Can you work these out from the model? Positions are in its coordinate system, mm. Round coordinates to 2 decimals unless told otherwise and drop trailing zeros. Loops run counter-clockwise (first coordinate to the right, second up) from the corner with the lowest first, then second, coordinate; pieces in that order, holes last. Notation, with made-up numbers: (42.25, 65.25) -> (63.25, 65.25) arc R12 ccw to (63.25, 81.25) -> close; hole circle Ø8 at (74.25, 36). An arc over 180 degrees is marked (long way). Use a Markdown table: item, result.
from build123d import *

# Parameters (mm, degrees)
SKETCH1_W           = 3.175
SKETCH1_H           = 7.62
BOSS_EXTRUDE1_DEPTH = 1.5875


with BuildPart() as part:
    # Sketch1 → Boss-Extrude1 (new body)
    with BuildSketch(Plane.XY):
        Polygon((232.626798958, 25.527772685), (-69.633201042, 22.867122461), (-69.633201042, 26.152979633), (-63.283201042, 26.152979633), (-63.283201042, 33.772979633), (-69.633201042, 33.772979633), (-69.633201042, 39.09426549), (232.626798958, 39.09426549), (232.626798958, 33.772979633), (229.451798958, 33.772979633), (229.451798958, 26.152979633), (232.626798958, 26.152979633), align=None)
        with Locations((158.649298958, 29.962979633)):
            Rectangle(SKETCH1_W, SKETCH1_H, mode=Mode.SUBTRACT)
        with Locations((83.084298958, 29.962979633)):
            Rectangle(SKETCH1_W, SKETCH1_H, mode=Mode.SUBTRACT)
        with Locations((7.519298958, 29.962979633)):
            Rectangle(SKETCH1_W, SKETCH1_H, mode=Mode.SUBTRACT)
    extrude(amount=BOSS_EXTRUDE1_DEPTH)


solid = part.part
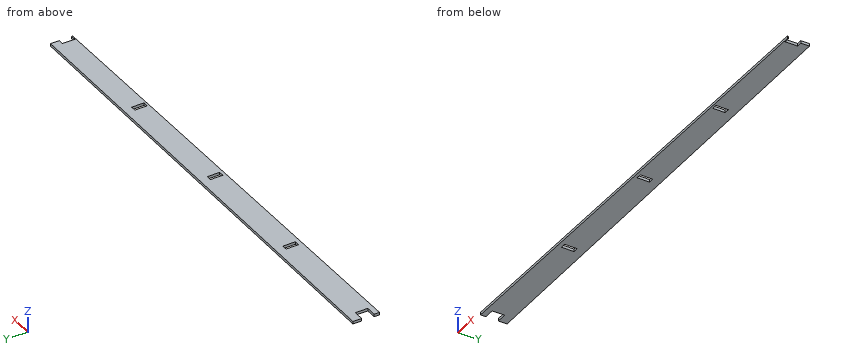
1. I want a section at D-D (x = -18.5). Please give me the cut outline in (y, z), plus the area to 3 significant figures.
Answer sheet:
| item | result |
|---|---|
| outline | (23.32, 0) -> (39.09, 0) -> (39.09, 1.59) -> (23.32, 1.59) -> close |
| area | 25.0 mm² |
2. I need wall thicknesses on line 1 (X direction, y = 33.25, z = 1.25); line 2 (Y direction, x = 201, z = 1.3); line 3 (Y direction, x = 149.5, z = 0.55). Which ranges of each line are inside material? Lowest first, please.
Answer sheet:
| item | result |
|---|---|
| line 1 | x = -63.28 to 5.93, 9.11 to 81.5, 84.67 to 157.06, 160.24 to 229.45 |
| line 2 | y = 25.25 to 39.09 |
| line 3 | y = 24.8 to 39.09 |
3. I want a section at B-B (z = 0.45). Please give me the cut outline in (x, y).
Answer sheet:
| item | result |
|---|---|
| outline | (-69.63, 22.87) -> (232.63, 25.53) -> (232.63, 26.15) -> (229.45, 26.15) -> (229.45, 33.77) -> (232.63, 33.77) -> (232.63, 39.09) -> (-69.63, 39.09) -> (-69.63, 33.77) -> (-63.28, 33.77) -> (-63.28, 26.15) -> (-69.63, 26.15) -> close; hole (5.93, 26.15) -> (9.11, 26.15) -> (9.11, 33.77) -> (5.93, 33.77) -> close; hole (81.5, 26.15) -> (84.67, 26.15) -> (84.67, 33.77) -> (81.5, 33.77) -> close; hole (157.06, 26.15) -> (160.24, 26.15) -> (160.24, 33.77) -> (157.06, 33.77) -> close |
4. I want a section at A-A (y = 30.25). Please give me the cut outline in (x, z), plus the area to 3 significant figures.
Answer sheet:
| item | result |
|---|---|
| outline | (-63.28, 0) -> (5.93, 0) -> (5.93, 1.59) -> (-63.28, 1.59) -> close; (9.11, 0) -> (81.5, 0) -> (81.5, 1.59) -> (9.11, 1.59) -> close; (84.67, 0) -> (157.06, 0) -> (157.06, 1.59) -> (84.67, 1.59) -> close; (160.24, 0) -> (229.45, 0) -> (229.45, 1.59) -> (160.24, 1.59) -> close |
| area | 450 mm² |
5. I want a section at C-C (x = 101). Please give me the cut outline in (y, z).
Answer sheet:
| item | result |
|---|---|
| outline | (24.37, 0) -> (39.09, 0) -> (39.09, 1.59) -> (24.37, 1.59) -> close |
6. Will these pins go through, and if not, where does the flat tip stop? pin 1 Ø0.5 at (x, z) = (158.5, 1) entering from -Y; pin 2 Ø0.5 at (y, z) = (29.5, 1) entering from +X; pin 3 Ø0.8 at (x, z) = (231, 1) entering from -Y.
Answer sheet:
| item | result |
|---|---|
| pin 1 | stops at y = 24.87 |
| pin 2 | stops at x = 229.45 |
| pin 3 | stops at y = 25.51 |
